```python
from build123d import *

# Parameters (mm, degrees)
F0_W      = 70.6123113632
F0_H      = 104.6859696507
F1_DEPTH  = 52.07
F2_R      = 20.6851974424
F3_DEPTH  = 118.618
F4_R      = 20.7250274732
F5_DEPTH  = 93.98
F6_DEPTH  = 21.59
F7_DEPTH  = 26.924
F8_DEPTH  = 13.208
F9_DEPTH  = 5.08
F10_DEPTH = 25.4


with BuildPart() as f1:
    # F0 (on Top) → F1 (new body)
    with BuildSketch(Plane.XY):
        Rectangle(F0_W, F0_H)
    extrude(amount=F1_DEPTH)

    # F2 (on face) → F3 (cut)
    with BuildSketch(Plane.XZ.offset(52.3429848254)):
        with Locations((-6.3621718436, 23.2127420604)):
            Circle(F2_R)
    extrude(amount=-F3_DEPTH, mode=Mode.SUBTRACT)

    # F4 (on face) → F5 (cut)
    with BuildSketch(Plane.YZ.offset(35.3061556816)):
        with Locations((2.8868210502, 23.3023613691)):
            Circle(F4_R)
    extrude(amount=-F5_DEPTH, mode=Mode.SUBTRACT)

    # F6 (cut): a face of the model
    f6_faces = [f1.faces().sort_by_distance(p)[0] for p in [
        (34.4288083492, 52.3429848254, 26.035),
    ]]
    extrude(f6_faces, amount=-F6_DEPTH, mode=Mode.SUBTRACT)

    # F7 (cut): a face of the model
    f7_faces = [f1.faces().sort_by_distance(p)[0] for p in [
        (-34.4288083492, -52.3429848254, 26.035),
    ]]
    extrude(f7_faces, amount=-F7_DEPTH, mode=Mode.SUBTRACT)

    # F8 (cut): a face of the model
    f8_faces = [f1.faces().sort_by_distance(p)[0] for p in [
        (35.3061556816, 2.667, 0.7659357071),
    ]]
    extrude(f8_faces, amount=-F8_DEPTH, mode=Mode.SUBTRACT)

    # F9 (cut): a face of the model
    f9_faces = [f1.faces().sort_by_distance(p)[0] for p in [
        (-6.604, 2.667, 52.07),
    ]]
    extrude(f9_faces, amount=-F9_DEPTH, mode=Mode.SUBTRACT)

    # F10 (intersect): a face of the model
    f10_faces = [f1.faces().sort_by_distance(p)[0] for p in [
        (22.0981556816, 2.667, 0.7323489793),
    ]]
    extrude(f10_faces, amount=-F10_DEPTH, mode=Mode.INTERSECT)


solid = f1.part
```
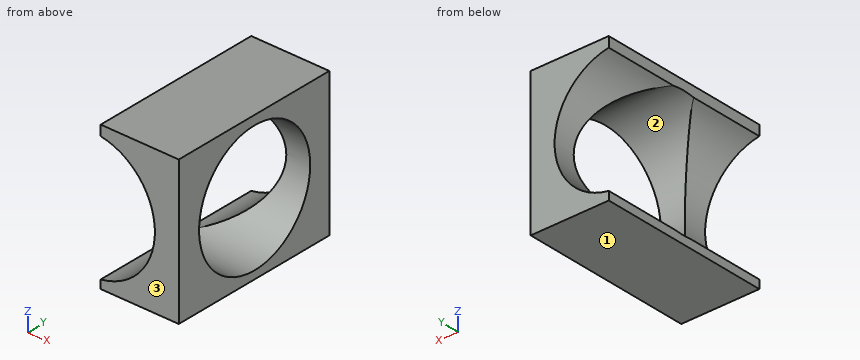
CAD build for the part. Positions are in the model's coordinates, mm. Face numbers are marked on the shaded views. Give positions to 0.01 mm unless a question says otherwise; leave off trailing zeros. Order: outer loops, then holes, each group sorted by start corner. A loop starts at its lowest first (then second) coordinate and runs counter-clockwise, first axis right, second up.
(1) Mould opens along Y. For the marked faces 1, 2 and 3 say: released by +Y, released by -Y, zero draft, split by the parting line, or undercut.
(2) Saw through at C-C, the plane y = 13.5. Give the cut face in (x, z), then the cut area to 3 significant figures.
(3) Saw through at B-B, the plane z = 13.5. Give the cut face in (x, y).
(4) Drill centre lines: L1, parallel to Z at x = 20, y = 2.5; L2, parallel to Y at x = 10.25, z = 5; L3, parallel to Y at x = 14.5, z = 5.5. Where is each one in solid material? Low to high.
(5) Saw through at D-D, the plane x = 10.5. Give the cut face in (y, z).
(6) Saw through at A-A, the plane x = 0. Give the cut face in (y, z), then the cut area to 3 significant figures.
Results found:
1. face 1: zero draft
1. face 2: undercut
1. face 3: released by -Y
2. outline: (-3.3, 0) - (22.1, 0) - (22.1, 5.5) - (4.32, 5.5) arc R20.69 cw to (-3.3, 2.76) - close; (-3.3, 43.67) arc R20.69 cw to (4.02, 41.1) - (22.1, 41.1) - (22.1, 46.99) - (-3.3, 46.99) - close
2. area: 265 mm2
3. outline: (11.9, -25.42) - (22.1, -25.42) - (22.1, -15.37) - (11.9, -15.37) - close; (11.9, 21.15) - (22.1, 21.15) - (22.1, 30.75) - (11.9, 30.75) - close
4. L1: z = 0 to 2.58, 44.02 to 46.99
4. L2: y = -25.42 to -6.84, 12.61 to 30.75
4. L3: y = -25.42 to -7.72, 13.5 to 30.75
5. outline: (-25.42, 0) - (30.75, 0) - (30.75, 11.23) - (19.73, 11.23) arc R20.73 cw to (-13.96, 11.23) - (-25.42, 11.23) - close; (-25.42, 35.19) - (-14.09, 35.19) arc R20.73 cw to (19.86, 35.19) - (30.75, 35.19) - (30.75, 46.99) - (-25.42, 46.99) - close
6. outline: (-25.42, 0) - (30.75, 0) - (30.75, 3.53) - (9.1, 3.53) arc R20.73 cw to (-3.33, 3.53) - (-25.42, 3.53) - close; (-25.42, 42.9) - (-3.87, 42.9) arc R20.73 cw to (9.64, 42.9) - (30.75, 42.9) - (30.75, 46.99) - (-25.42, 46.99) - close
6. area: 410 mm2
